```python
from build123d import *

# Parameters (mm, degrees)
F0_W     = 22.225
F0_H     = 101.6
F1_DEPTH = 6.35
F2_W     = 12.7
F2_H     = 3.175
F3_DEPTH = 3.175
F4_SIZE  = 2.54


# Not quite as in the source:
# - a pattern or mirror of a feature is missing from the dataset's text; its kind, count and spacing are read off the source's solid


with BuildPart() as f1:
    # F0 (on Top) → F1 (new body)
    with BuildSketch(Plane.XY):
        Rectangle(F0_W, F0_H)
    extrude(amount=F1_DEPTH)

    # F2 (on face) → F3 (join)
    with BuildSketch(Plane.YZ.offset(11.1125)):
        with Locations((-41.275, 1.5875)):
            Rectangle(F2_W, F2_H)
        with Locations((0, 1.5875)):
            Rectangle(F2_W, F2_H)
        with Locations((41.275, 1.5875)):
            Rectangle(F2_W, F2_H)
    f3 = extrude(amount=F3_DEPTH)

    # F3_copies: F3 across plane
    add(f3.mirror(Plane(origin=(0, 0, 0), x_dir=(0, 0, -1), z_dir=(-1, 0, 0))))

    # F4
    f4_edges = [f1.edges().sort_by_distance(p)[0] for p in [
        (0, 50.8, 6.35),
        (0, -50.8, 6.35),
    ]]
    chamfer(f4_edges, length=F4_SIZE)


solid = f1.part
```
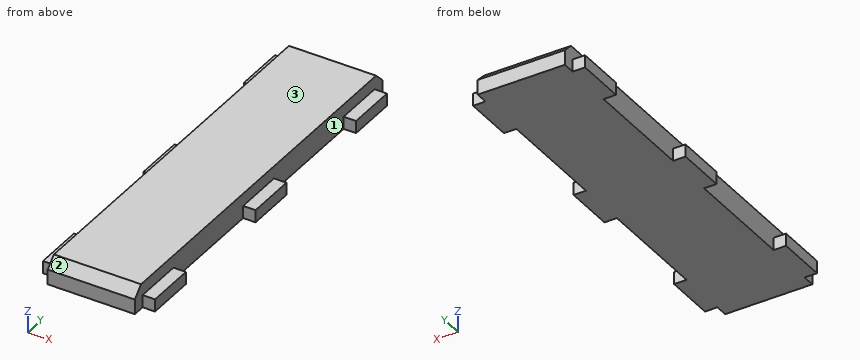
CAD build for the part. Positions are in the model's coordinates, mm. Face numbers are marked on the shaded views. Coordinates: 2 decimals unless noted, no trailing zeros. Loops run counter-clockwise (first coordinate to the right, second up) from the corner with the lowest first, then second, coordinate; pieces in that order, holes last. Notation, with made-up numbers: (-31.5, 87) - (-5.5, 87) arc R35 cw to (-5.5, 125) - close; hole circle Ø8 at (20, 58). An arc over 180 degrees is marked (long way). Return JSON: item names as keys, results as strings.
1. Drop flat-ended pins along their axis: pin 1 (1.6 mm diameter, centred on x = 12, z = 1, fed in from +Y) (3 decimals); pin 2 (1.6 mm diameter, centred on x = -12, z = 1.5, fed in from -Y) (3 decimals); pin 3 (2.5 mm diameter, centred on x = -13, y = 41.5, fed in from +Z) (3 decimals). Give the stop position or say it passes through.
Result:
{"pin 1": "stops at y = 47.625", "pin 2": "stops at y = -47.625", "pin 3": "stops at z = 3.175"}
2. Mould opens along Y. For the marked faces 1, 2 and 3 say: released by +Y, released by -Y, zero draft, split by the parting line, or undercut.
Result:
{"face 1": "undercut", "face 2": "released by -Y", "face 3": "zero draft"}
3. Probe L1, parallel to X at y = 14, z = 4.5; L2, parallel to Y at x = 10.5, z = 5.75; L3, parallel to Y at x = -4.25, z = 4.25. List the from-to ranges inside material, lowest first. Write a range as from..to.
Result:
{"L1": "x = -11.11..11.11", "L2": "y = -48.86..48.86", "L3": "y = -50.36..50.36"}
4. Band-saw the part on C-C (y = 26.5). Give the cut face in (x, z).
Result:
{"outline": "(-11.11, 0) - (11.11, 0) - (11.11, 6.35) - (-11.11, 6.35) - close"}
